Part model, mm, in its own coordinate system. Face numbers are marked on the shaded views. A direction names the side the tool comes from. Give positions to 0.01 mm unless a question says otherwise; leave off trailing zeros. Order: outer loops, then holes, each group sorted by start corner. A loop starts at its lowest first (then second) coordinate and runs counter-clockwise, first axis right, second up. Notation, with made-up numbers: (85.25, -2) - (96.25, -2) arc R24 ccw to (96.25, 24) - close; hole circle Ø11 at (-11, 26). An arc over 180 degrees is marked (long way). Use one line per item in the form item = value. Start each with the question number.
1. Tool access for the marked faces 4 and 5: list every direction of +Z, -Z, +X, -X, +Y, -Y with a clear straight run to the whole face (end or side of a thin tool).
2. Band-saw the part on A-A, the plane y = 92.5. List the corners of the cut face in (x, z), plus the area to 3 significant figures.
3. Band-saw the part on C-C, the plane z = -90.5. List the corners of the cut face in (x, y), plus the area to 3 significant figures.
4. Pin check, flat tips, straight feed: P1, Ø2.5, axis at y = 14.5, z = -101.5, coming from the +X side; P2, Ø8, axis at y = 20, z = -92, coming from the -X side; P3, Ø5.5, axis at x = -38.1, y = 67.1, coming from the +Z side; P4, Ø6, axis at x = -24, z = -92.5, coming from the -Y side. Stop position of each tip, or through.
5. Drill centre lines: line 1 (Y direction, x = 30, z = -105); line 2 (X direction, y = 57.5, z = -95); line 3 (X direction, y = 87, z = -107.75). Where is each one in solid material? Low to high.
6. Pull direction X, two halves, no side cores. Call the marked faces 1, 2 and 3: +X half, -X half, draft (parallel to the pull), parting line (faces both ways), or undercut.
7. Band-saw the part on D-D, the plane x = -2. List the corners of the cut face in (y, z), plus the area to 3 significant figures.
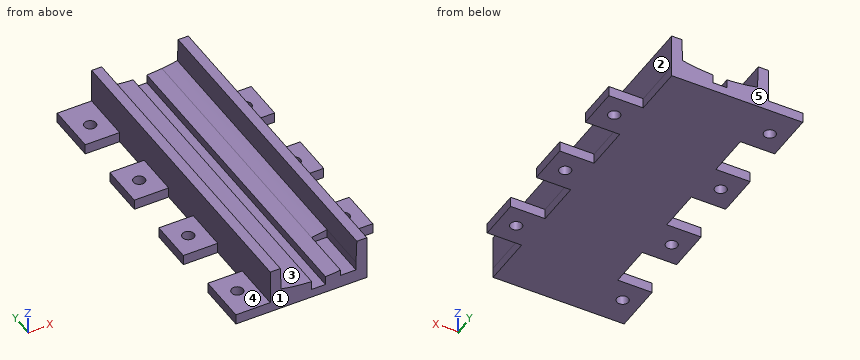
from build123d import *

# Parameters (mm, degrees)
F1_DEPTH = 185
F3_DEPTH = 30
F2_W     = 10
F2_H     = 12.7
F2_W_2   = 20
F2_H_2   = 29.6450595204
F2_H_3   = 26.5
F2_H_4   = 30.8181657076
F4_DEPTH = 25
F5_D     = 6.7564


# Not quite as in the source:
# - a feature names something its author has since deleted; it is built from what else it names


with BuildPart() as f1:
    # F0 (on Front) → F1 (new body)
    with BuildSketch(Plane.XZ):
        with BuildLine():
            Line((-28.0998, -84.153), (-28.0998, -96.0750292217))
            ThreePointArc((-28.0998, -96.0750292217), (-24.948943425, -96.9410141373), (-21.7715, -97.7036938286))
            Line((-21.7715, -97.7036938286), (-22.2458, -84.153))
            Line((-22.2458, -84.153), (-28.0998, -84.153))
        make_face()
        with BuildLine():
            ThreePointArc((-21.7715, -97.7036938286), (-24.948943425, -96.9410141373), (-28.0998, -96.0750292217))
            Line((-28.0998, -96.0750292217), (-28.0998, -104.153))
            Line((-28.0998, -104.153), (-48.0998, -104.153))
            Line((-48.0998, -104.153), (-48.0998, -110.153))
            Line((-48.0998, -110.153), (0, -110.153))
            Line((0, -110.153), (48.0998, -110.153))
            Line((48.0998, -110.153), (48.0998, -104.153))
            Line((48.0998, -104.153), (28.0998, -104.153))
            Line((28.0998, -104.153), (28.0998, -96.0750292217))
            ThreePointArc((28.0998, -96.0750292217), (24.948943425, -96.9410141373), (21.7715, -97.7036938286))
            Line((21.7715, -97.7036938286), (21.7715, -102.7036938286))
            Line((21.7715, -102.7036938286), (12.7715, -102.7036938286))
            Line((12.7715, -102.7036938286), (12.7715, -99.2819157135))
            ThreePointArc((12.7715, -99.2819157135), (8.3938675756, -99.747446018), (4, -100.0200479904))
            Line((4, -100.0200479904), (4, -105.1526938286))
            Line((4, -105.1526938286), (-4, -105.1526938286))
            Line((-4, -105.1526938286), (-4, -100.0200479904))
            ThreePointArc((-4, -100.0200479904), (-12.9376940454, -99.2603952883), (-21.7715, -97.7036938286))
        make_face()
        with BuildLine():
            ThreePointArc((21.7715, -97.7036938286), (24.948943425, -96.9410141373), (28.0998, -96.0750292217))
            Line((28.0998, -96.0750292217), (28.0998, -84.153))
            Line((28.0998, -84.153), (22.2458, -84.153))
            Line((22.2458, -84.153), (21.7715, -97.7036938286))
        make_face()
        with BuildLine():
            Line((21.7715, -102.7036938286), (21.7715, -97.7036938286))
            ThreePointArc((21.7715, -97.7036938286), (17.289517296, -98.5955505673), (12.7715, -99.2819157135))
            Line((12.7715, -99.2819157135), (12.7715, -102.7036938286))
            Line((12.7715, -102.7036938286), (21.7715, -102.7036938286))
        make_face()
    extrude(amount=-F1_DEPTH)

    # F0 (on Front) → F3 (cut)
    with BuildSketch(Plane.XZ):
        with BuildLine():
            Line((21.7715, -102.7036938286), (21.7715, -97.7036938286))
            ThreePointArc((21.7715, -97.7036938286), (17.289517296, -98.5955505673), (12.7715, -99.2819157135))
            Line((12.7715, -99.2819157135), (12.7715, -102.7036938286))
            Line((12.7715, -102.7036938286), (21.7715, -102.7036938286))
        make_face()
    extrude(amount=-F3_DEPTH, mode=Mode.SUBTRACT)

    # F2 (on face) → F4 (cut)
    with BuildSketch(Plane.XY.offset(-104.153)):
        Polygon((-48.0998, 29), (-38.0998, 29), (-38.0998, 41.7), (-38.0998, 54.4), (-48.0998, 54.4), align=None)
        with Locations((-33.0998, 35.35)):
            Rectangle(F2_W, F2_H)
        Polygon((-48.0998, 105.2), (-48.0998, 79.8), (-38.0998, 79.8), (-38.0998, 92.5), (-38.0998, 105.2), align=None)
        with Locations((-33.0998, 86.15)):
            Rectangle(F2_W, F2_H)
        Polygon((-48.0998, 156), (-48.0998, 130.6), (-38.0998, 130.6), (-38.0998, 143.3), (-38.0998, 156), align=None)
        with Locations((-33.0998, 136.95)):
            Rectangle(F2_W, F2_H)
        with Locations((-33.0998, 48.05)):
            Rectangle(F2_W, F2_H)
        with Locations((-33.0998, 98.85)):
            Rectangle(F2_W, F2_H)
        with Locations((-33.0998, 149.65)):
            Rectangle(F2_W, F2_H)
        with Locations((38.1002, 14.7274702398)):
            Rectangle(F2_W_2, F2_H_2)
        with Locations((38.1002, 67.1)):
            Rectangle(F2_W_2, F2_H_3)
        with Locations((38.1002, 117.9)):
            Rectangle(F2_W_2, F2_H_3)
        with Locations((38.1002, 170.8590828538)):
            Rectangle(F2_W_2, F2_H_4)
    extrude(amount=-F4_DEPTH, mode=Mode.SUBTRACT)

    # F5 (through all)
    with Locations(Plane.XY.offset(-104.153)):
        with Locations((-38.0998, 67.1), (-38.0998, 16.3), (-38.0998, 117.9), (-38.0998, 168.7), (38.1002, 92.5), (38.1002, 143.3), (38.1002, 41.7)):
            Hole(F5_D / 2)


solid = f1.part
From the geometry:
q1.face_4 = +Z, -X, +Y, -Y
q1.face_5 = +Z, -Z, +X, -X, +Y
q2.outline = (-28.1, -110.15) - (34.72, -110.15) - (34.72, -104.15) - (28.1, -104.15) - (28.1, -84.15) - (22.25, -84.15) - (21.77, -97.7) arc R100.1 cw to (4, -100.02) - (4, -105.15) - (-4, -105.15) - (-4, -100.02) arc R100.1 cw to (-21.77, -97.7) - (-22.25, -84.15) - (-28.1, -84.15) - close; (41.48, -110.15) - (48.1, -110.15) - (48.1, -104.15) - (41.48, -104.15) - close
q2.area = 834 mm²
q3.outline = (-28.1, 0) - (-22.02, 0) - (-22.02, 185) - (-28.1, 185) - close; (22.02, 0) - (28.1, 0) - (28.1, 185) - (22.02, 185) - close
q3.area = 2,250 mm²
q4.P1 = 28.1
q4.P2 = -28.1
q4.P3 = through
q4.P4 = 0
q5.line_1 = 29.55 to 53.85, 80.35 to 104.65, 131.15 to 155.45
q5.line_2 = -28.1 to -21.87, 21.87 to 28.1
q5.line_3 = -28.1 to 48.1
q6.face_1 = draft
q6.face_2 = +X half
q6.face_3 = undercut
q7.outline = (0, -110.15) - (185, -110.15) - (185, -105.15) - (0, -105.15) - close
q7.area = 925 mm²
